```python
from build123d import *

# Parameters (mm, degrees)
P_IDAT_VYSUNUT_M1_DEPTH = 2.4


with BuildPart() as part:
    # Skica1 → Přidat vysunutím1 (new body)
    with BuildSketch(Plane(origin=(0, 0, 0), x_dir=(1, 0, 0), z_dir=(0, 1, 0))):
        Polygon((41.3, 87.4), (41.3, 85), (-2.4, 85), (-2.4, 43.7), (0, 43.7), (0, 0), (41.3, 0), (41.3, 2.4), (85, 2.4), (85, 43.7), (82.6, 43.7), (82.6, 87.4), align=None)
    extrude(amount=P_IDAT_VYSUNUT_M1_DEPTH)


solid = part.part
```
Design review of the part built by this model. Coordinates are the model's own, in mm. A direction names the side the tool comes from. Coordinates: 2 decimals unless noted, no trailing zeros. Write each loop counter-clockwise with the first axis right and the second up, starting at its lowest first coordinate (ties: lowest second). Pieces come first, ordered by that corner, then holes. Notation, with made-up numbers: M 82.25,-26 L 120.25,-26 A11 ccw 120.25,-7 Z; hole C 66,87.5 d1. An arc over 180 degrees is marked long. Answer as a JSON object with one key per item and string values.
Item 1: Insertion check: pin 1 Ø1.2 at (x, y) = (-1, 1) entering from +Z; pin 2 Ø0.7 at (y, z) = (0.5, -23.5) entering from -X; pin 3 Ø0.7 at (x, y) = (84, 1.5) entering from -Z. Each pin has a flat end and moves straight along its axis. Give the tip position at first contact, or say it passes through.
Outcome:
{"pin 1": "z = -43.7", "pin 2": "x = 0", "pin 3": "z = -43.7"}
Item 2: Machinability: for faces 1 (the flat face through (20, 1, -85)), 2 (the flat face through (-1, 1, -43.7)), 3 (the flat face through (84, 1, -43.7)), 4 (the flat face through (41.3, 1, -1)), which of the approach directions +Z, -Z, +X, -X, +Y, -Y give a long, thin tool a straight path to every point of the face, cutting with its end or side? Answer none if there is none.
Outcome:
{"face 1": "-Z, -X, +Y, -Y", "face 2": "+Z, -X, +Y, -Y", "face 3": "-Z, +X, +Y, -Y", "face 4": "+Z, +X, +Y, -Y"}
Item 3: Add section C-C, the plane z = -72.5. Give the boundary of the cut face in (x, y), and give its area (3 significant figures).
Outcome:
{"outline": "M -2.4,0 L 82.6,0 L 82.6,2.4 L -2.4,2.4 Z", "area": "204 mm²"}
Item 4: Add section B-B, the plane x = 66.5. Give the boundary of the cut face in (y, z), and give its area (3 significant figures).
Outcome:
{"outline": "M 0,-87.4 L 2.4,-87.4 L 2.4,-2.4 L 0,-2.4 Z", "area": "204 mm²"}
Item 5: Wall thickness on probe 1 along Z at (x, y) = (58.5, 1.35); probe 2 along X at (y, z) = (1.4, -24); probe 3 along X at (y, z) = (2.1, -82): over which ranges is each line inside the solid? List them lowest first.
Outcome:
{"probe 1": "-87.4 to -2.4", "probe 2": "0 to 85", "probe 3": "-2.4 to 82.6"}
Item 6: Add section A-A, the plane y = 1.5. Give the boundary of the cut face in (x, z), and give its area (3 significant figures).
Outcome:
{"outline": "M -2.4,-85 L 41.3,-85 L 41.3,-87.4 L 82.6,-87.4 L 82.6,-43.7 L 85,-43.7 L 85,-2.4 L 41.3,-2.4 L 41.3,0 L 0,0 L 0,-43.7 L -2.4,-43.7 Z", "area": "7,220 mm²"}
